The listing builds one solid part. Answer for the finished solid, in the listing's coordinates (mm). A direction names the side the tool comes from. Round coordinates to 2 decimals unless told otherwise and drop trailing zeros. Order: outer loops, then holes, each group sorted by start corner. A loop starts at its lowest first (then second) coordinate and runs counter-clockwise, first axis right, second up. Notation, with made-up numbers: (79.25, 8.5) - (92.25, 8.5) arc R31 cw to (92.25, 32.5) - close; hole circle Ø3 at (-26.75, 44.25). An arc over 180 degrees is marked (long way). One line per item, written item: value. Start each with the question number.
1. For a pull along Y with two mould halves and no side action, classify faces 1 (the cylindrical face through (-1.08, -4.88, 2.46)), 2 (the flat face through (-1, 7, 0)), 3 (the flat face through (1, 30, 4)) as released by +Y, released by -Y, zero draft, split by the parting line, or undercut.
2. Straight lines are drawn through the part: line 1 (X direction, y = 12, z = 32.5); line 2 (Y direction, x = 0, z = 2.2); line 3 (Z direction, x = 34.5, y = 12). For each, find the intervals that lie inside material, in ascending order.
3. Section D-D, the plane y = -11 is taken. Give the vertices of the cut face in (x, z).
4. Section C-C, the plane x = 0 is taken. Give the vertices of the cut face in (y, z), then the cut area to 3 significant figures.
5. A tool of negligible diameter and unlimited length cuts with its end or side. For faces 4 (the flat face through (-35, 0, 46)), 5 (the flat face through (1, -30, 4)), from which of +Z, -Z, +X, -X, +Y, -Y can it reach the whole face along a straight path? Write none if from no direction.
6. Section B-B, the plane y = 0 is taken. Give the vertices of the cut face in (x, z), then the cut area to 3 significant figures.
7. Flat-ended cylindrical pins translate along their axes: P1, Ø18, axis at x = 5, y = 10, coming from the +Z side; P2, Ø10, axis at y = 11, z = 73, coming from the -X side (3 decimals); P3, Ø2, axis at y = -20.5, z = 75, coming from the -X side (3 decimals). Find the tip coordinate at first contact, or state that the pin passes through.
8. Section A-A, the plane z = 40 is taken. Give the vertices of the cut face in (x, y).
from build123d import *

# Parameters (mm, degrees)
SKETCH1_W           = 150
SKETCH1_H           = 60
SKETCH1_R           = 5
BOSS_EXTRUDE1_DEPTH = 5
BOSS_EXTRUDE2_DEPTH = 60


with BuildPart() as part:
    # Sketch1 → Boss-Extrude1 (new body)
    with BuildSketch(Plane.XY):
        Rectangle(SKETCH1_W, SKETCH1_H)
        Circle(SKETCH1_R, mode=Mode.SUBTRACT)
    extrude(amount=BOSS_EXTRUDE1_DEPTH)

    # Sketch2 → Boss-Extrude2 (add)
    with BuildSketch(Plane(origin=(0, 30, 0), x_dir=(1, 0, 0), z_dir=(0, 1, 0))):
        Polygon((-35, -85), (-35, -5), (-75, -5), (-75, -45), (-60, -85), align=None)
    boss_extrude2 = extrude(amount=-BOSS_EXTRUDE2_DEPTH)

    # Mirror1: Boss-Extrude2 across plane
    add(boss_extrude2.mirror(Plane(origin=(0, 0, 0), x_dir=(0, 0, 1), z_dir=(1, 0, 0))))


solid = part.part
Answer list:
1. face 1: undercut
1. face 2: zero draft
1. face 3: released by +Y
2. line 1: x = -75 to -35, 35 to 75
2. line 2: y = -30 to -5, 5 to 30
2. line 3: z = 0 to 5
3. outline: (-75, 0) - (75, 0) - (75, 45) - (60, 85) - (35, 85) - (35, 5) - (-35, 5) - (-35, 85) - (-60, 85) - (-75, 45) - close
4. outline: (-30, 0) - (-5, 0) - (-5, 5) - (-30, 5) - close; (5, 0) - (30, 0) - (30, 5) - (5, 5) - close
4. area: 250 mm²
5. face 4: +Z, +Y, -Y
5. face 5: +Z, -Z, +X, -X, -Y
6. outline: (-75, 0) - (-5, 0) - (-5, 5) - (-35, 5) - (-35, 85) - (-60, 85) - (-75, 45) - close; (5, 0) - (75, 0) - (75, 45) - (60, 85) - (35, 85) - (35, 5) - (5, 5) - close
6. area: 6,500 mm²
7. P1: stops at z = 5
7. P2: stops at x = -66.375
7. P3: stops at x = -64.125
8. outline: (-75, -30) - (-35, -30) - (-35, 30) - (-75, 30) - close; (35, -30) - (75, -30) - (75, 30) - (35, 30) - close
